Build history of the part. All positions in model axes, mm. A direction names the side the tool comes from. Give positions to 0.01 mm unless a question says otherwise; leave off trailing zeros. Write each loop counter-clockwise with the first axis right and the second up, starting at its lowest first coordinate (ties: lowest second). Pieces come first, ordered by that corner, then holes. Notation, with made-up numbers: (12.25, 89) -> (45.25, 89) arc R19 cw to (45.25, 110) -> close; hole circle Ø4 at (57, 5.5). An arc over 180 degrees is marked (long way). Write item = value, one per line. Start each with the question number.
Q1. Tool access for faces 5 (the face through (52, 15, -1)), 6 (the face through (-1, 3, 18)): list every direction of +Z, -Z, +X, -X, +Y, -Y with a clear straight run to the whole face (end or side of a thin tool).
Q2. Drop flat-ended pins along their axis: P1, Ø5, axis at x = 42.5, z = 16, coming from the +Y side; P2, Ø3.5, axis at x = 43.55, z = -28, coming from the +Y side; P3, Ø1.3, axis at x = 46.5, y = 2, coming from the +Z side. Give the stop position or say it passes through.
Q3. Mould opens along X. For faces 1 (the face through (1, 15, 52)), 2 (the face through (39, 3, 4)), 3 (the face through (46, 6, 4)), 4 (the face through (50, 14.8, 49.9)) say: pulls with the +X half, pulls with the -X half, needs draft (parallel to the pull), parting line crosses it, or undercut.
Q4. Saw through at C-C, the plane x = -32.5. List the corners of the cut face in (y, z), then the cut area to 3 significant figures.
Q5. Saw through at B-B, the plane y = 11. List the corners of the cut face in (x, z).
Q6. Wall check: line 1 (X direction, y = 3, z = 15); line 2 (X direction, y = 3.4, z = 4); line 3 (Z direction, x = -2.5, y = 2.5). Give the ranges that are in metal, low to high.
Q7. Saw through at A-A, the plane z = 21.5. List the corners of the cut face in (x, y), then the cut area to 3 significant figures.
Q8. Saw through at D-D, the plane z = 4. List the corners of the cut face in (x, y).
from build123d import *

# Parameters (mm, degrees)
BOSS_EXTRUDE1_DEPTH = 32
SHELL1_T            = 2
SKETCH2_R           = 2.05
SKETCH2_W           = 100
SKETCH2_H           = 6
BOSS_EXTRUDE2_DEPTH = 6
FILLET1_R           = 2
SKETCH3_W           = 11.15
SKETCH3_H           = 6
BOSS_EXTRUDE3_DEPTH = 1.6
SKETCH4_R           = 2.05
CUT_EXTRUDE1_DEPTH  = 7.6


with BuildPart() as part:
    # Sketch1 → Boss-Extrude1 (new body)
    with BuildSketch(Plane(origin=(0, 0, 0), x_dir=(1, 0, 0), z_dir=(0, 1, 0))):
        with BuildLine():
            Line((-45, 50), (45, 50))
            ThreePointArc((45, 50), (48.535533906, 48.535533906), (50, 45))
            Line((50, 45), (50, -45))
            ThreePointArc((50, -45), (48.535533906, -48.535533906), (45, -50))
            Line((45, -50), (-45, -50))
            ThreePointArc((-45, -50), (-48.535533906, -48.535533906), (-50, -45))
            Line((-50, -45), (-50, 45))
            ThreePointArc((-50, 45), (-48.535533906, 48.535533906), (-45, 50))
        make_face()
    extrude(amount=BOSS_EXTRUDE1_DEPTH)

    # Shell1
    shell1_openings = [part.faces().sort_by_distance(p)[0] for p in [
        (0, 32, 0),
    ]]
    offset(amount=SHELL1_T, openings=shell1_openings, kind=Kind.INTERSECTION)

    # Sketch2 → Boss-Extrude2 (add)
    # profile 1 of 5: a face of its own
    with BuildSketch(Plane(origin=(0, 0, 0), x_dir=(1, 0, 0), z_dir=(0, 1, 0))):
        with BuildLine():
            Line((-43.55, 32.55), (-50, 32.55))
            Line((-50, 32.55), (-50, 23.45))
            Line((-50, 23.45), (-43.55, 23.45))
            ThreePointArc((-43.55, 23.45), (-39, 28), (-43.55, 32.55))
        make_face()
        with Locations(Location((-43.55, 28, 0), (0, 0, 270))):
            Circle(SKETCH2_R, mode=Mode.SUBTRACT)
    # profile 2 of 5: a face of its own
    with BuildSketch(Plane(origin=(0, 0, 0), x_dir=(1, 0, 0), z_dir=(0, 1, 0))):
        with BuildLine():
            Line((-43.55, 0.55), (-50, 0.55))
            Line((-50, 0.55), (-50, -8.55))
            Line((-50, -8.55), (-43.55, -8.55))
            ThreePointArc((-43.55, -8.55), (-39, -4), (-43.55, 0.55))
        make_face()
        with Locations(Location((-43.55, -4, 0), (0, 0, 270))):
            Circle(SKETCH2_R, mode=Mode.SUBTRACT)
    # profile 3 of 5: a face of its own
    with BuildSketch(Plane(origin=(0, 0, 0), x_dir=(1, 0, 0), z_dir=(0, 1, 0))):
        with BuildLine():
            Line((43.55, 0.55), (50, 0.55))
            Line((50, 0.55), (50, -8.55))
            Line((50, -8.55), (43.55, -8.55))
            ThreePointArc((43.55, -8.55), (39, -4), (43.55, 0.55))
        make_face()
        with Locations(Location((43.55, -4, 0), (0, 0, 270))):
            Circle(SKETCH2_R, mode=Mode.SUBTRACT)
    # profile 4 of 5: a face of its own
    with BuildSketch(Plane(origin=(0, 0, 0), x_dir=(1, 0, 0), z_dir=(0, 1, 0))):
        with BuildLine():
            Line((43.55, 32.55), (50, 32.55))
            Line((50, 32.55), (50, 23.45))
            Line((50, 23.45), (43.55, 23.45))
            ThreePointArc((43.55, 23.45), (39, 28), (43.55, 32.55))
        make_face()
        with Locations(Location((43.55, 28, 0), (0, 0, 270))):
            Circle(SKETCH2_R, mode=Mode.SUBTRACT)
    # profile 5 of 5: a face of its own
    with BuildSketch(Plane(origin=(0, 0, 0), x_dir=(1, 0, 0), z_dir=(0, 1, 0))):
        with Locations((0, -15)):
            Rectangle(SKETCH2_W, SKETCH2_H)
    extrude(amount=BOSS_EXTRUDE2_DEPTH)

    # Fillet1
    fillet1_edges = [part.edges().sort_by_distance(p)[0] for p in [
        (50, 3, 8.55),
        (50, 3, -0.55),
        (50, 3, -23.45),
        (50, 3, -32.55),
        (-50, 3, -23.45),
        (-50, 3, -32.55),
        (-50, 3, -0.55),
        (-50, 3, 8.55),
    ]]
    fillet(fillet1_edges, radius=FILLET1_R)

    # Sketch3 → Boss-Extrude3 (add)
    with BuildSketch(Plane(origin=(0, 6, 0), x_dir=(1, 0, 0), z_dir=(0, 1, 0))):
        with Locations((-44.425, -15)):
            Rectangle(SKETCH3_W, SKETCH3_H)
        with Locations((44.425, -15)):
            Rectangle(SKETCH3_W, SKETCH3_H)
    extrude(amount=BOSS_EXTRUDE3_DEPTH)

    # Sketch4 → Cut-Extrude1 (cut)
    with BuildSketch(Plane(origin=(0, 7.6, 0), x_dir=(1, 0, 0), z_dir=(0, 1, 0))):
        with Locations(Location((-43.55, -15, 0), (0, 0, 270))):
            Circle(SKETCH4_R)
        with Locations(Location((43.55, -15, 0), (0, 0, 270))):
            Circle(SKETCH4_R)
    extrude(amount=-CUT_EXTRUDE1_DEPTH, mode=Mode.SUBTRACT)


solid = part.part
Report:
q1.face_5 = +Z, -Z, +X, +Y, -Y
q1.face_6 = +Y
q2.P1 = 7.6
q2.P2 = 0
q2.P3 = 51.95
q3.face_1 = needs draft
q3.face_2 = undercut
q3.face_3 = undercut
q3.face_4 = pulls with the +X half
q4.outline = (-2, -52) -> (32, -52) -> (32, -50) -> (0, -50) -> (0, 12) -> (6, 12) -> (6, 18) -> (0, 18) -> (0, 50) -> (32, 50) -> (32, 52) -> (-2, 52) -> close
q4.area = 372 mm2
q5.outline = (-52, -45) arc R7 ccw to (-45, -52) -> (45, -52) arc R7 ccw to (52, -45) -> (52, 45) arc R7 ccw to (45, 52) -> (-45, 52) arc R7 ccw to (-52, 45) -> close; hole (-50, -45) arc R5 ccw to (-45, -50) -> (45, -50) arc R5 ccw to (50, -45) -> (50, 45) arc R5 ccw to (45, 50) -> (-45, 50) arc R5 ccw to (-50, 45) -> close
q6.line_1 = -52 to -45.6, -41.5 to 41.5, 45.6 to 52
q6.line_2 = -52 to -45.6, -41.5 to -39, 39 to 41.5, 45.6 to 52
q6.line_3 = -52 to -50, 12 to 18, 50 to 52
q7.outline = (-52, -2) -> (52, -2) -> (52, 32) -> (50, 32) -> (50, 0) -> (-50, 0) -> (-50, 32) -> (-52, 32) -> close
q7.area = 336 mm2
q8.outline = (-52, -2) -> (52, -2) -> (52, 32) -> (50, 32) -> (50, 6) -> (45.6, 6) -> (45.6, 0) -> (41.5, 0) -> (41.5, 6) -> (39, 6) -> (39, 0) -> (-39, 0) -> (-39, 6) -> (-41.5, 6) -> (-41.5, 0) -> (-45.6, 0) -> (-45.6, 6) -> (-50, 6) -> (-50, 32) -> (-52, 32) -> close
